The listing builds one solid part. Answer for the finished solid, in the listing's coordinates (mm). Round coordinates to 2 decimals unless told otherwise and drop trailing zeros. Write each loop counter-clockwise with the first axis right and the second up, starting at its lowest first coordinate (ties: lowest second). Pieces come first, ordered by that corner, then holes. Notation, with made-up numbers: (-8, 72.25) - (16, 72.25) arc R8 cw to (16, 77.25) - close; hole circle Ø11 at (-0.75, 22.5). An arc over 180 degrees is marked (long way). Use a Markdown table: item, result. Add a question column.
1) Find the intervals of material crossed by probe 1 along Z at (x, y) = (0, 7.5); probe 2 along X at (y, z) = (1.5, -0.5); probe 3 along X at (y, z) = (4.25, -58), in increasing order. Write a range as from..to.
2) A cutting plane is placed at C-C (y = 8). State how many separate pieces and enclosed holes the cut face has, then the cut area to 3 significant figures.
3) A cutting plane is placed at B-B (z = 0). Give the vertices of the cut face in (x, y) (3 decimals), then the cut area to 3 significant figures.
4) A cutting plane is placed at A-A (x = 0). Give the vertices of the cut face in (y, z) (3 decimals).
5) A cutting plane is placed at D-D (z = -46). Give the vertices of the cut face in (x, y) (1 decimal).
6) Each of these flat-tipped pins is pushed along its axis until it touches: P1, Ø1.5, axis at x = 86, y = 3, coming from the -Z side; P2, Ø5.5, axis at x = -102.84, z = -59.37, coming from the -Y side; P3, Ø4, axis at x = 85.5, y = 4.5, coming from the +Z side; P4, Ø19, axis at x = -36.5, z = -27.5, coming from the -Y side. Where does it stop, or does it pass through?
```python
from build123d import *

# Parameters (mm, degrees)
SKETCH1_W               = 127
SKETCH1_H               = 9.525
F_1_4_CLEARANCE_HOLE1_D = 6.7564
CUT_EXTRUDE1_REACH      = 181.858
SKETCH4_W               = 50.8
SKETCH4_H               = 2.565921067
CUT_EXTRUDE2_REACH      = 181.858
SKETCH6_R               = 16.51
SKETCH7_R               = 19
CUT_EXTRUDE3_DEPTH      = 2


with BuildPart() as part:
    # Sketch1 → Revolve1 (revolve)
    with BuildSketch(Plane.XY, mode=Mode.PRIVATE) as revolve1_sk:
        with Locations((63.5, 4.7625)):
            Rectangle(SKETCH1_W, SKETCH1_H)
    revolve(revolve1_sk.sketch.rotate(Axis((0, 0, 0), (0, 1, 0)), 90), axis=Axis((0, 0, 0), (0, 1, 0)))

    # 1/4 Clearance Hole1 (through all)
    with Locations(Plane(origin=(0, 9.525, 0), x_dir=(1, 0, 0), z_dir=(0, 1, 0))):
        with Locations((0, 118.745), (59.3725, 102.836186572), (102.836186572, 59.3725), (118.745, 0), (102.836186572, -59.3725), (59.3725, -102.836186572), (0, -118.745), (-59.3725, -102.836186572), (-102.836186572, -59.3725), (-118.745, 0), (-102.836186572, 59.3725), (-59.3725, 102.836186572)):
            Hole(F_1_4_CLEARANCE_HOLE1_D / 2)

    # Sketch4 → Cut-Extrude1 (cut, up to next)
    with BuildSketch(Plane(origin=(0, 9.525, 0), x_dir=(1, 0, 0), z_dir=(0, 1, 0)), mode=Mode.PRIVATE) as cut_extrude1_sk1:
        with Locations((0, -125.717039467)):
            Rectangle(SKETCH4_W, SKETCH4_H)
    cut_extrude1_tool1 = extrude(cut_extrude1_sk1.sketch, amount=-CUT_EXTRUDE1_REACH, mode=Mode.PRIVATE) & part.part
    add(cut_extrude1_tool1.solids().sort_by_distance((0, 9.525, 125.717039))[0], mode=Mode.SUBTRACT)

    # Sketch6 → Cut-Extrude2 (cut, up to next)
    with BuildSketch(Plane.XZ, mode=Mode.PRIVATE) as cut_extrude2_sk1:
        with Locations(Location((-35.921024484, -35.921024484, 0), (0, 0, 270))):
            Circle(SKETCH6_R)
    cut_extrude2_tool1 = extrude(cut_extrude2_sk1.sketch, amount=-CUT_EXTRUDE2_REACH, mode=Mode.PRIVATE) & part.part
    add(cut_extrude2_tool1.solids().sort_by_distance((-35.921024, 0, -35.921024))[0], mode=Mode.SUBTRACT)

    # Sketch7 → Cut-Extrude3 (cut)
    with BuildSketch(Plane.XZ):
        with Locations(Location((-35.921024484, -35.921024484, 0), (0, 0, 270))):
            Circle(SKETCH7_R)
    extrude(amount=-CUT_EXTRUDE3_DEPTH, mode=Mode.SUBTRACT)


solid = part.part
```
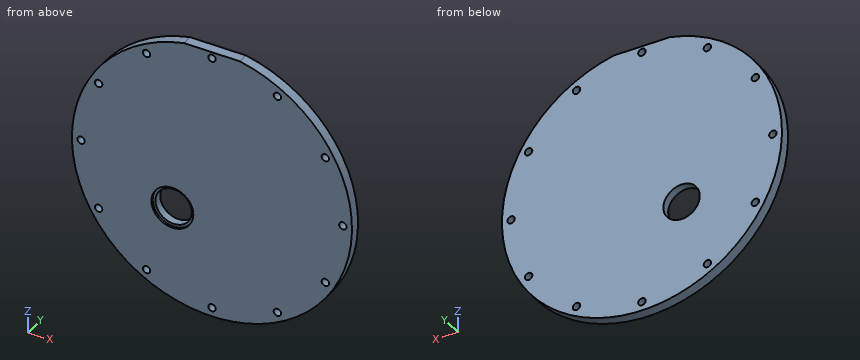
Entries:
| question | item | result |
|---|---|---|
| 1 | probe 1 | z = -127..-122.12, -115.37..115.37, 122.12..124.43 |
| 1 | probe 2 | x = -127..-122.09, -115.4..115.4, 122.09..127 |
| 1 | probe 3 | x = -112.98..-105.92, -99.75..99.75, 105.92..112.98 |
| 2 | separate pieces | 1 |
| 2 | enclosed holes | 13 |
| 2 | area | 49,300 mm² |
| 3 | outline | (-127, 0) - (-122.123, 0) - (-122.123, 9.525) - (-127, 9.525) - close; (-115.367, 0) - (115.367, 0) - (115.367, 9.525) - (-115.367, 9.525) - close; (122.123, 0) - (127, 0) - (127, 9.525) - (122.123, 9.525) - close |
| 3 | area | 2,290 mm² |
| 4 | outline | (0, -127) - (9.525, -127) - (9.525, -122.123) - (0, -122.123) - close; (0, -115.367) - (9.525, -115.367) - (9.525, 115.367) - (0, 115.367) - close; (0, 122.123) - (9.525, 122.123) - (9.525, 124.434) - (0, 124.434) - close |
| 5 | outline | (-118.4, 0) - (-52, 0) - (-52, 2) - (-49, 2) - (-49, 9.5) - (-118.4, 9.5) - close; (-22.8, 2) - (-19.8, 2) - (-19.8, 0) - (118.4, 0) - (118.4, 9.5) - (-22.8, 9.5) - close |
| 6 | P1 | stops at z = -94.14 |
| 6 | P2 | passes through |
| 6 | P3 | stops at z = 95.69 |
| 6 | P4 | stops at y = 2 |
